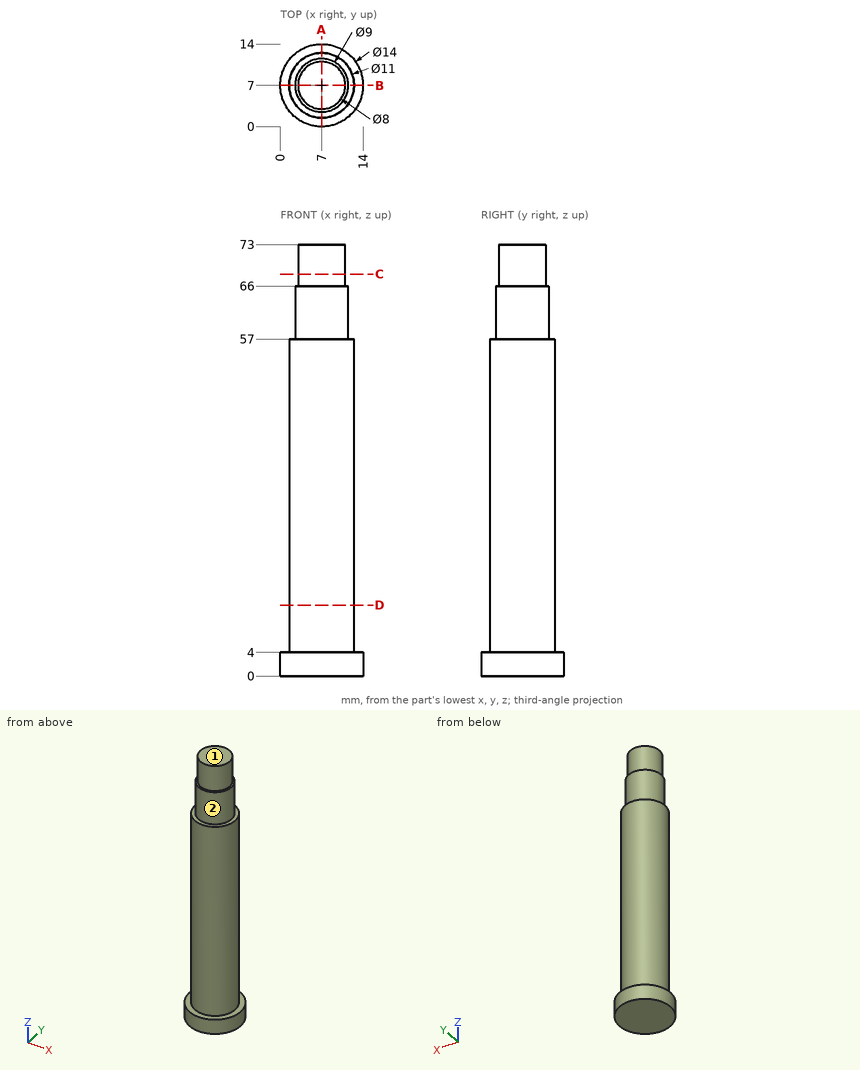
Study the drawing (mm; zero at the part's minimum x, y, z) and answer. A direction names the side the tool comes from. Give positions to 0.01 mm unless a question says otherwise; leave off trailing zeros. Loops run counter-clockwise (first coordinate to the right, second up) from the corner with the lowest first, then second, coordinate; pieces in that order, holes last. Notation, with made-up numbers: (81.25, -9.75) - (100.25, -9.75) arc R10 ccw to (100.25, -5.75) - close; hole circle Ø8 at (35, 64.5). An arc over 180 degrees is marked (long way). Answer in a Markdown table with one row per item. Add a question column.
Q1. Each of these flat-tipped pins is pushed along its axis until it touches: P1, Ø5, axis at x = 9.5, z = 22, coming from the -Y side; P2, Ø2, axis at x = 11, z = 44, coming from the -Y side; P3, Ø1, axis at y = 8.5, z = 30.5, coming from the +X side. Where does it stop, or does it pass through?
Q2. The part is cut by section D-D (z = 12). Determine the outline of the cut face in (x, y).
Q3. Consider line 1 along Y through (x, z) = (6.75, 7.5); line 2 along Z through (x, y) = (4, 11.75); line 3 along Z through (x, y) = (2.25, 6.75). Determine where each line is inside the solid, lowest interval first.
Q4. The part is cut by section A-A (x = 7). Determine the outline of the cut face in (y, z), and give its area (3 significant figures).
Q5. A tool of negligible diameter and unlimited length cuts with its end or side. For the marked faces 1 and 2, from which of +Z, -Z, +X, -X, +Y, -Y can it reach the whole face along a straight path? Write none if from no direction.
Q6. The part is cut by section C-C (z = 68). Determine the outline of the cut face in (x, y).
Solution:
| question | item | result |
|---|---|---|
| 1 | P1 | stops at y = 1.5 |
| 1 | P2 | stops at y = 2.39 |
| 1 | P3 | stops at x = 12.41 |
| 2 | outline | circle Ø11 at (7, 7) |
| 3 | line 1 | y = 1.51 to 12.49 |
| 3 | line 2 | z = 0 to 4 |
| 3 | line 3 | z = 0 to 57 |
| 4 | outline | (0, 0) - (14, 0) - (14, 4) - (12.5, 4) - (12.5, 57) - (11.5, 57) - (11.5, 66) - (11, 66) - (11, 73) - (3, 73) - (3, 66) - (2.5, 66) - (2.5, 57) - (1.5, 57) - (1.5, 4) - (0, 4) - close |
| 4 | area | 776 mm² |
| 5 | face 1 | +Z, +X, -X, +Y, -Y |
| 5 | face 2 | +Z |
| 6 | outline | circle Ø8 at (7, 7) |
